Build history of the part. All positions in model axes, mm. A direction names the side the tool comes from. Give positions to 0.01 mm unless a question says otherwise; leave off trailing zeros. Order: outer loops, then holes, each group sorted by start corner. A loop starts at its lowest first (then second) coordinate and runs counter-clockwise, first axis right, second up. Notation, with made-up numbers: (-7.75, 64.5) -> (44.25, 64.5) arc R19 ccw to (44.25, 80.5) -> close; hole circle Ø5 at (60, -16). An arc over 180 degrees is marked (long way). One line per item, written item: value. Start each with the question number.
(1) Saw through at C-C on z = -17. Give the cut face in (x, y) (1 decimal), plus the area to 3 significant figures.
(2) Saw through at D-D on x = 0. Give the cut face in (y, z) (1 decimal).
(3) Two-plate mould, pull along Z, no slides. Class faces 4 (the flat face through (-3, 9.525, 15)), 5 (the flat face through (-3, 6, 19.844)), 6 (the flat face through (-3, 6, -19.844)), 7 (the cylindrical face through (56.184, 0.805, 25.934)): +Z half, -Z half, draft (parallel to the pull), parting line (faces both ways), or undercut.
(4) Saw through at B-B on x = 57.15. Give the cut face in (y, z).
(5) Probe line 1 (Z direction, x = 57.15, y = 0.5); line 2 (Y direction, x = -42, z = 27); line 3 (Z direction, x = 2, y = 4.5). List the from-to ranges inside material, lowest first.
(6) Which spindle directions (+Z, -Z, +X, -X, +Y, -Y) get a long thin tool onto all of the face, cutting with end or side? Do faces 1 (the flat face through (-3, 6, -10.319)), 2 (the flat face through (-15.081, 6, -15)), 3 (the flat face through (10.319, 6, -15)). Say none if no direction does.
(7) Pin check, flat tips, straight feed: pin 1 (2.5 mm diameter, centred on x = 2, y = 7, fed in from +Z); pin 2 (5 mm diameter, centred on x = 8.5, z = 11, fed in from -Y); pin 3 (4.5 mm diameter, centred on x = 57.15, z = 26.99, fed in from +Y); pin 4 (4 mm diameter, centred on x = -5, y = 4, fed in from -Z). Stop position of each tip, or through.
(8) Saw through at A-A on y = 3.75. Give the cut face in (x, z), plus the area to 3 significant figures.
```python
from build123d import *

# Parameters (mm, degrees)
SKETCH1_W                                  = 119.0625
SKETCH1_H                                  = 58.7375
BOSS_EXTRUDE1_DEPTH                        = 1.5875
SKETCH2_W                                  = 25.4
SKETCH2_H                                  = 9.525
BOSS_EXTRUDE2_DEPTH                        = 7.9375
SKETCH3_R                                  = 1.42875
CUT_EXTRUDE1_DEPTH                         = 67.854297613
MIRROR2_AT_THE_SECOND_PLANE_COPY_1_SKETC_R = 1.42875
MIRROR2_AT_THE_SECOND_PLANE_COPY_1_DEPTH   = 67.854297613


with BuildPart() as part:
    # Sketch1 → Boss-Extrude1 (new body)
    with BuildSketch(Plane(origin=(0, 0, 0), x_dir=(1, 0, 0), z_dir=(0, 1, 0))):
        Rectangle(SKETCH1_W, SKETCH1_H)
    extrude(amount=BOSS_EXTRUDE1_DEPTH)

    # Sketch2 → Boss-Extrude2 (add)
    with BuildSketch(Plane(origin=(0, 1.5875, 0), x_dir=(1, 0, 0), z_dir=(0, 1, 0))):
        with Locations((-2.38125, -15.08125)):
            Rectangle(SKETCH2_W, SKETCH2_H)
    boss_extrude2 = extrude(amount=BOSS_EXTRUDE2_DEPTH)

    # Mirror1: Boss-Extrude2 across plane
    add(boss_extrude2.mirror(Plane.XY))

    # Sketch3 → Cut-Extrude1 (cut, through all)
    with BuildSketch(Plane(origin=(0, 1.5875, 0), x_dir=(1, 0, 0), z_dir=(0, 1, 0))):
        with Locations(Location((-57.15, -26.9875, 0), (0, 0, 270))):
            Circle(SKETCH3_R)
    cut_extrude1 = extrude(amount=-CUT_EXTRUDE1_DEPTH, mode=Mode.SUBTRACT)

    # Mirror2: Cut-Extrude1 across plane
    add(cut_extrude1.mirror(Plane(origin=(0, 0, 0), x_dir=(0, 0, 1), z_dir=(1, 0, 0))), mode=Mode.SUBTRACT)

    # Mirror2 at the second plane: Cut-Extrude1 across plane
    add(cut_extrude1.mirror(Plane.XY), mode=Mode.SUBTRACT)

    # Mirror2 at the second plane copy 1 sketc → Mirror2 at the second plane copy 1 (cut, through all)
    with BuildSketch(Plane(origin=(0, 1.5875, 0), x_dir=(-1, 0, 0), z_dir=(0, 1, 0))):
        with Locations(Location((-57.15, -26.9875, 0), (0, 0, 270))):
            Circle(MIRROR2_AT_THE_SECOND_PLANE_COPY_1_SKETC_R)
    extrude(amount=-MIRROR2_AT_THE_SECOND_PLANE_COPY_1_DEPTH, mode=Mode.SUBTRACT)


solid = part.part
```
Results below:
1. outline: (-59.5, 0) -> (59.5, 0) -> (59.5, 1.6) -> (10.3, 1.6) -> (10.3, 9.5) -> (-15.1, 9.5) -> (-15.1, 1.6) -> (-59.5, 1.6) -> close
1. area: 391 mm²
2. outline: (0, -29.4) -> (1.6, -29.4) -> (1.6, -19.8) -> (9.5, -19.8) -> (9.5, -10.3) -> (1.6, -10.3) -> (1.6, 10.3) -> (9.5, 10.3) -> (9.5, 19.8) -> (1.6, 19.8) -> (1.6, 29.4) -> (0, 29.4) -> close
3. face 4: draft
3. face 5: +Z half
3. face 6: -Z half
3. face 7: undercut
4. outline: (0, -29.37) -> (1.59, -29.37) -> (1.59, -28.42) -> (0, -28.42) -> close; (0, -25.56) -> (1.59, -25.56) -> (1.59, 25.56) -> (0, 25.56) -> close; (0, 28.42) -> (1.59, 28.42) -> (1.59, 29.37) -> (0, 29.37) -> close
5. line 1: z = -29.37 to -28.42, -25.56 to 25.56, 28.42 to 29.37
5. line 2: y = 0 to 1.59
5. line 3: z = -19.84 to -10.32, 10.32 to 19.84
6. face 1: +X, -X, +Y
6. face 2: +Z, -Z, -X, +Y
6. face 3: +Z, -Z, +X, +Y
7. pin 1: stops at z = 19.84
7. pin 2: stops at y = 0
7. pin 3: stops at y = 1.59
7. pin 4: stops at z = -19.84
8. outline: (-15.08, -19.84) -> (10.32, -19.84) -> (10.32, -10.32) -> (-15.08, -10.32) -> close; (-15.08, 10.32) -> (10.32, 10.32) -> (10.32, 19.84) -> (-15.08, 19.84) -> close
8. area: 484 mm²
